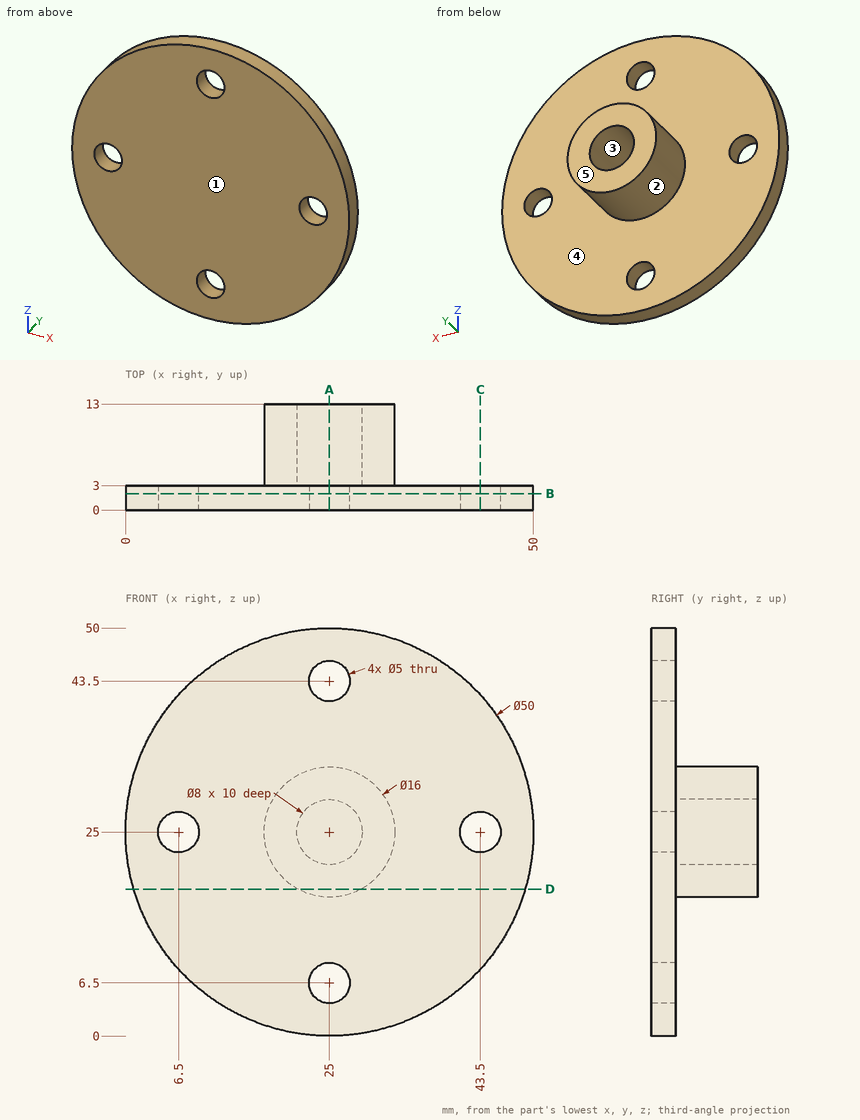
Source: three-view drawing plus pictorial views. Frame: mm from the lowest corner of the part. A direction names the side the tool comes from. Give positions to 0.01 mm unless a question says otherwise; leave off trailing zeros. Order: outer loops, then holes, each group sorted by start corner. A loop starts at its lowest first (then second) coordinate and runs counter-clockwise, first axis right, second up. Notation, with made-up numbers: M -0.5,27 L 54.5,27 A29 cw 54.5,52 Z; hole C 59.5,85.25 d8. An arc over 180 degrees is marked long. Return JSON: item names as keys, results as strings.
Item 1: Cut plane D-D (z = 18). Return loops of the section in (x, y).
Solutions:
{"outline": "M 1,0 L 49,0 L 49,3 L 28.87,3 L 28.87,13 L 21.13,13 L 21.13,3 L 1,3 Z"}
Item 2: Ray query, probe 1 along X at (y, z) = (1.15, 25); probe 2 along Z at (x, y) = (25, 10.5). Return the intervals inside material, ascending.
Solutions:
{"probe 1": "0 to 4, 9 to 41, 46 to 50", "probe 2": "17 to 21, 29 to 33"}
Item 3: Cut plane A-A (x = 25). Return loops of the section in (y, z).
Solutions:
{"outline": "M 0,0 L 3,0 L 3,4 L 0,4 Z; M 0,9 L 3,9 L 3,17 L 13,17 L 13,21 L 3,21 L 3,29 L 13,29 L 13,33 L 3,33 L 3,41 L 0,41 Z; M 0,46 L 3,46 L 3,50 L 0,50 Z"}
Item 4: Access query for the marked faces 4 and 5. Directions: +Z, -Z, +X, -X, +Y, -Y. A direction counts if a zero-diameter tool reaches every point of the face in a straight line with its end or side. Return the directions, or none.
Solutions:
{"face 4": "+Y", "face 5": "+Z, -Z, +X, -X, +Y"}
Item 5: Cut plane B-B (y = 2). Return loops of the section in (x, z), then the cut area to 3 significant figures.
Solutions:
{"outline": "C 25,25 d50; hole C 6.5,25 d5; hole C 25,6.5 d5; hole C 25,43.5 d5; hole C 43.5,25 d5", "area": "1,880 mm^2"}
Item 6: Cut plane C-C (x = 43.5). Return loops of the section in (y, z), then the cut area to 3 significant figures.
Solutions:
{"outline": "M 0,8.18 L 3,8.18 L 3,22.5 L 0,22.5 Z; M 0,27.5 L 3,27.5 L 3,41.82 L 0,41.82 Z", "area": "85.9 mm^2"}
Item 7: Pull-direction query (Z, two-part tool) for the marked faces 1, 2 and 3; classes: +Z half, -Z half, draft (parallel to the pull), parting line (faces both ways), or undercut.
Solutions:
{"face 1": "draft", "face 2": "parting line", "face 3": "undercut"}
Item 8: First-contact query: P1, Ø6.5, axis at x = 6.5, z = 25, coming from the +Y side; P2, Ø4, axis at x = 43.5, z = 25, coming from the -Y side; P3, Ø6, axis at y = 4.5, z = 31.5, coming from the -X side; P4, Ø1, axis at x = 30.5, y = 7.5, coming from the +Z side (3 decimals). Flat tips, straight axial feed; report the tip coordinate or a pass-through.
Solutions:
{"P1": "y = 3", "P2": "through", "P3": "x = 0.31", "P4": "z = 31.245"}
